from build123d import *

# Parameters (mm, degrees)
F0_W      = 13.49375
F0_H      = 19.05
F1_DEPTH  = 241.3
F2_W      = 3.96875
F2_H      = 9.525
F3_DEPTH  = 19.051
F5_DEPTH  = 13.49475
F6_SIZE   = 6.35
F9_W      = 3.175
F9_H      = 431.8
F10_DEPTH = 6.35


with BuildPart() as f1:
    # F0 (on Front) → F1 (new body)
    with BuildSketch(Plane.XZ):
        with Locations((-6.746875, 9.525)):
            Rectangle(F0_W, F0_H)
    extrude(amount=F1_DEPTH)

    # F2 (on Top) → F3 (cut, through all)
    with BuildSketch(Plane.XY):
        with Locations((-11.509375, -220.6625)):
            Rectangle(F2_W, F2_H)
    extrude(amount=F3_DEPTH, mode=Mode.SUBTRACT)

    # F4 (on Right) → F5 (cut, through all)
    with BuildSketch(Plane.YZ):
        Polygon((-215.9, 0), (-215.9, 6.35), (-225.425, 6.35), (-241.3, 7.9375), (-241.3, 0), align=None)
    extrude(amount=-F5_DEPTH, mode=Mode.SUBTRACT)

    # F6
    f6_edges = [f1.edges().sort_by_distance(p)[0] for p in [
        (-13.49375, -241.3, 13.49375),
    ]]
    chamfer(f6_edges, length=F6_SIZE)

    # F7: F1 across plane


with BuildPart() as f1_1:
    add(f1.part)
    add(f1.part.mirror(Plane.YZ))

    # F8: F1 across plane


with BuildPart() as f1_2:
    add(f1_1.part)
    add(f1_1.part.mirror(Plane.XZ))

    # F9 (on face) → F10 (cut)
    with BuildSketch(Plane(origin=(0, 0, 0), x_dir=(1, 0, 0), z_dir=(0, 0, -1))):
        Rectangle(F9_W, F9_H)
    extrude(amount=-F10_DEPTH, mode=Mode.SUBTRACT)


solid = f1_2.part
Build history of the part. All positions in model axes, mm. A direction names the side the tool comes from. Coordinates: 2 decimals unless noted, no trailing zeros. Order: outer loops, then holes, each group sorted by start corner. A loop starts at its lowest first (then second) coordinate and runs counter-clockwise, first axis right, second up. Notation, with made-up numbers: (-19, 3) - (-7, 3) arc R15 ccw to (-7, 13) - close; hole circle Ø8 at (-3, -14). An arc over 180 degrees is marked (long way). Put each result on its own line as item: value.
1. Tool access for faces 1 (the face through (-10, -215.9, 7)), 2 (the face through (-9.525, -221, 13)), 3 (the face through (9.525, 221, 13)): list every direction of +Z, -Z, +X, -X, +Y, -Y with a clear straight run to the whole face (end or side of a thin tool).
Answer sheet:
face 1: -Z, -X
face 2: +Z, -Z, -X
face 3: +Z, -Z, +X
2. Probe line 1 along X through (y, z) = (-206, 4.5); line 2 along Y through (x, z) = (-3, 1.25); line 3 along Y through (x, z) = (-12, 14.25) (3 decimals). List the from-to ranges inside material, lowest first. Write a range as [from, to].
Answer sheet:
line 1: x = [-13.49, -1.59], [1.59, 13.49]
line 2: y = [-215.9, 215.9]
line 3: y = [-236.444, -225.425], [-215.9, 215.9], [225.425, 236.444]
3. Saw through at A-A (y = -156.5). Write the cut outline in (x, z).
Answer sheet:
outline: (-13.49, 0) - (-1.59, 0) - (-1.59, 6.35) - (1.59, 6.35) - (1.59, 0) - (13.49, 0) - (13.49, 19.05) - (-13.49, 19.05) - close
4. Pull direction X, two halves, no side cores. Call faces 4 (the face through (-1, -1, 6.35)), 5 (the face through (9.525, -221, 13)), 6 (the face through (-7, -3, 0)): pulls with the +X half, pulls with the -X half, needs draft (parallel to the pull), parting line crosses it, or undercut.
Answer sheet:
face 4: undercut
face 5: pulls with the +X half
face 6: needs draft
5. Saw through at B-B (z = 14). Write the cut outline in (x, y) (3 decimals), and give its area (3 significant figures).
Answer sheet:
outline: (-13.494, -234.95) - (-7.144, -241.3) - (7.144, -241.3) - (13.494, -234.95) - (13.494, -225.425) - (9.525, -225.425) - (9.525, -215.9) - (13.494, -215.9) - (13.494, 215.9) - (9.525, 215.9) - (9.525, 225.425) - (13.494, 225.425) - (13.494, 234.95) - (7.144, 241.3) - (-7.144, 241.3) - (-13.494, 234.95) - (-13.494, 225.425) - (-9.525, 225.425) - (-9.525, 215.9) - (-13.494, 215.9) - (-13.494, -215.9) - (-9.525, -215.9) - (-9.525, -225.425) - (-13.494, -225.425) - close
area: 12,800 mm^2
6. Drop flat-ended pins along their axis: P1, Ø2, axis at x = -12.5, z = 10, coming from the +Y side; P2, Ø1.5, axis at x = 8.5, z = 3, coming from the -Y side; P3, Ø3, axis at x = -11, z = 11, coming from the -Y side. Give the stop position or say it passes through.
Answer sheet:
P1: stops at y = 236.94
P2: stops at y = -215.9
P3: stops at y = -238.94
